Autodesk Inventor part; units mm, degrees
ref_plane "YZ Plane" through (0, 0, 0) normal (1, 0, 0) x (0, 1, 0)
ref_plane "XZ Plane" through (0, 0, 0) normal (0, 1, 0) x (-1, 0, 0)
ref_plane "XY Plane" through (0, 0, 0) normal (0, 0, 1) x (1, 0, 0)
sketch "Boceto1" plane through (0, 0, 0) normal (0, 0, 1) x (1, 0, 0)
  circle A0 centre (0, 0) radius 1.75
  circle A1 centre (0, 0) radius 9.25
  line L0 (43, 17) -> (-96.75, 17)
  line L1 (-9.25, 0) -> (-9.25, 17)
  line L2 (9.25, 0) -> (9.25, 17)
  dimension "d0" = 3.5
  dimension "d1" = 18.5
extrude "Extrusión1" add sketch "Boceto1" along normal blind 2
ref_plane "Plano de trabajo1" through (83.25, 17, -70.5) normal (0, -1, 0) x (1, 0, 0)
sketch "Boceto3" plane through (83.25, 17, -70.5) normal (0, -1, 0) x (1, 0, 0)
  line L0 (-74, 72.5) -> (-92.5, 72.5)
  line L1 (-92.5, 72.5) -> (-74, 72.5)
  line L2 (-74, 72.5) -> (-74, 79.5)
  line L3 (-74, 79.5) -> (-92.5, 79.5)
  line L4 (-92.5, 79.5) -> (-92.5, 72.5)
  line L5 (-74, 76) -> (-78, 76)
  circle A0 centre (-78, 76) radius 1.5
  line L6 (-92.5, 76) -> (-88.5, 76)
  circle A1 centre (-88.5, 76) radius 1.5
  point P0 (-83.25, 70.5)
  dimension "d4" = 7
  dimension "d5" = 4
  dimension "d6" = 3
  dimension "d7" = 4
  dimension "d8" = 3
extrude "Extrusión2" add sketch "Boceto3" along normal blind 2
fillet "Empalme1" radius 2 1 edges at (0, 15, 2)
properties part number "Soporte Motor"
Design review of the part built by this model. Coordinates are the model's own, in mm. A direction names the side the tool comes from. Give positions to 0.01 mm unless a question says otherwise; leave off trailing zeros. Order: outer loops, then holes, each group sorted by start corner. A loop starts at its lowest first (then second) coordinate and runs counter-clockwise, first axis right, second up. Notation, with made-up numbers: (-31.75, 38) - (23.25, 38) arc R20 ccw to (23.25, 65) - close; hole circle Ø11 at (-4, 27.5). An arc over 180 degrees is marked (long way). Use a Markdown table: item, result. Add a question column.
(1) Machinability: for faces 5 (the face through (9.25, 10.4, 1.8)), 6 (the face through (0, 2, 2)), which of the approach directions +Z, -Z, +X, -X, +Y, -Y give a long, thin tool a straight path to every point of the face, cutting with its end or side? Answer none if there is none.
(2) Clearance check with flat-ended pins moving along their axes: P1, Ø3.5, axis at x = -5.25, z = 5.5, coming from the +Y side; P2, Ø6, axis at x = 6.5, y = -5.5, coming from the +Z side; P3, Ø4, axis at x = -3, y = 11.5, coming from the +Z side; P4, Ø1, axis at x = 6.5, z = 3, coming from the -Y side. State where each tip first meets the part, or that it passes through.
(3) Wall thickness on probe 1 along Y at (x, z) = (0, 0.45); probe 2 along Z at (x, y) = (5.25, 15.9); probe 3 along Y at (x, z) = (2.5, 5.75): over which ranges is each line inside the solid? List them lowest first. Write a range as [from, to].
(4) Add section C-C on x = -3. Give the boundary of the cut face in (y, z).
(5) Add section B-B on x = -5.75. Give the boundary of the cut face in (y, z), then the cut area to 3 significant figures.
(6) Add section A-A on z = 5.5. Give the boundary of the cut face in (x, y), then the cut area to 3 significant figures.
(7) Add section D-D on z = 1.5. Give the boundary of the cut face in (x, y).
(8) Mouldability with a two-part tool opening along Z and no side actions: class faces 1 (the face through (0, 4, 0)), 2 (the face through (-0.13, 14.43, 2.6)), 3 (the face through (6.056, 16.014, 4.235)), 4 (the face through (-9.25, 9.8, 1.5)) as +Z half, -Z half, draft (parallel to the pull), parting line (faces both ways), or undercut.
Report:
| question | item | result |
|---|---|---|
| 1 | face 5 | +Z, -Z, +X, +Y, -Y |
| 1 | face 6 | +Z, +X, -X, -Y |
| 2 | P1 | stops at y = 17 |
| 2 | P2 | stops at z = 2 |
| 2 | P3 | stops at z = 2.06 |
| 2 | P4 | stops at y = 14.32 |
| 3 | probe 1 | y = [-9.25, -1.75], [1.75, 17] |
| 3 | probe 2 | z = [0, 4], [7, 9] |
| 3 | probe 3 | y = [15, 17] |
| 4 | outline | (-8.75, 0) - (17, 0) - (17, 9) - (15, 9) - (15, 4) arc R2 cw to (13, 2) - (-8.75, 2) - close |
| 5 | outline | (-7.25, 0) - (17, 0) - (17, 4.09) - (15, 4.09) - (15, 4) arc R2 cw to (13, 2) - (-7.25, 2) - close; (15, 6.91) - (17, 6.91) - (17, 9) - (15, 9) - close |
| 5 | area | 57.7 mm² |
| 6 | outline | (-9.25, 15) - (-6.75, 15) - (-6.75, 17) - (-9.25, 17) - close; (-3.75, 15) - (3.75, 15) - (3.75, 17) - (-3.75, 17) - close; (6.75, 15) - (9.25, 15) - (9.25, 17) - (6.75, 17) - close |
| 6 | area | 25.0 mm² |
| 7 | outline | (-9.25, 0) arc R9.25 ccw to (9.25, 0) - (9.25, 17) - (-9.25, 17) - close; hole circle Ø3.5 at (0, 0) |
| 8 | face 1 | -Z half |
| 8 | face 2 | +Z half |
| 8 | face 3 | undercut |
| 8 | face 4 | draft |
